```python
from build123d import *

# Parameters (mm, degrees)
EXTRUDE_1_DEPTH = 5
SKETCH_2_W      = 20
SKETCH_2_H      = 40
EXTRUDE_3_DEPTH = 15
FILLET_1_R      = 10


with BuildPart() as part:
    # 草图1 → 凸台-拉伸1 (new body)
    with BuildSketch(Plane(origin=(0, 0, 0), x_dir=(1, 0, 0), z_dir=(0, 1, 0))):
        with BuildLine():
            Line((0, 0), (100, 0))
            Line((100, 0), (100, 112))
            Line((100, 112), (70, 152))
            ThreePointArc((70, 152), (50, 162), (30, 152))
            Line((30, 152), (0, 112))
            Line((0, 112), (0, 0))
        make_face()
    extrude(amount=EXTRUDE_1_DEPTH)

    # 草图2 → 凸台-拉伸3 (add)
    with BuildSketch(Plane.XZ):
        with Locations((90, -20)):
            Rectangle(SKETCH_2_W, SKETCH_2_H)
        with Locations((10, -20)):
            Rectangle(SKETCH_2_W, SKETCH_2_H)
    extrude(amount=EXTRUDE_3_DEPTH)

    # 圆角1
    fillet_1_edges = [part.edges().sort_by_distance(p)[0] for p in [
        (90, -15, 0),
        (10, -15, 0),
    ]]
    fillet(fillet_1_edges, radius=FILLET_1_R)


solid = part.part
```
Here's how the part is built. I have some questions about the finished solid (model axes, mm). A direction names the side the tool comes from. Round coordinates to 2 decimals unless told otherwise and drop trailing zeros. Order: outer loops, then holes, each group sorted by start corner. A loop starts at its lowest first (then second) coordinate and runs counter-clockwise, first axis right, second up. Notation, with made-up numbers: M -20.75,59.25 L -10.75,59.25 A24 ccw -10.75,71.25 Z; hole C 30,77 d10. An arc over 180 degrees is marked long. Answer as CSV lines item,"result".
Item 1: Please list where these lines run through material, in increasing order: L1, parallel to X at y = -13.75, z = -15.5; L2, parallel to Y at x = 64, z = -69; L3, parallel to Z at x = 88, y = -1. Write a range as [from, to].
From the geometry:
L1,"[0, 20], [80, 100]"
L2,"[0, 5]"
L3,"[-40, 0]"
Item 2: Imagine slicing it at C-C on z = -125. List the corners of the cut face in (x, y) for me.
From the geometry:
outline,"M 9.75,0 L 90.25,0 L 90.25,5 L 9.75,5 Z"
Item 3: Which directions (+Z, -Z, +X, -X, +Y, -Y) give clear straight access to the entire face, cutting with the end or side of a thin tool? Please do faces 1 (the flat face through (0, -3, -32)), 2 (the flat face through (10, -7, -40)), 3 (the flat face through (20, -7, -20)).
From the geometry:
face 1,"+Z, -Z, -X, +Y, -Y"
face 2,"-Z, +X, -X, -Y"
face 3,"+Z, -Z, -Y"
Item 4: Imagine slicing it at A-A on y = -1.75. List the corners of the cut face in (x, z) for me.
From the geometry:
outline,"M 0,-40 L 20,-40 L 20,0 L 0,0 Z; M 80,-40 L 100,-40 L 100,0 L 80,0 Z"
Item 5: We'd pull the mould along X, two halves only. Please class faces 4 (the flat face through (100, -3, -32)), 5 (the flat face through (80, -7, -20)), 6 (the cylindrical face through (90.14, -12.15, -3.01)): +X half, -X half, draft (parallel to the pull), parting line (faces both ways), or undercut.
From the geometry:
face 4,"+X half"
face 5,"undercut"
face 6,"draft"
Item 6: For pin 1 (10 mm diameter, centred on x = 12, y = -0.5, fed in from -Z); pin 2 (7.5 mm diameter, centred on x = 9.5, y = -8, fed in from -Z); pin 3 (6 mm diameter, centred on x = 72.5, y = 1, fed in from +Z), each with a flat end and sliding along its axis, tell me the tip position at first contact or that it passes through.
From the geometry:
pin 1,"z = -134.63"
pin 2,"z = -40"
pin 3,"z = 0"
Item 7: Imagine slicing it at D-D on y = -10. List the corners of the cut face in (x, z) for me.
From the geometry:
outline,"M 0,-40 L 20,-40 L 20,-1.34 L 0,-1.34 Z; M 80,-40 L 100,-40 L 100,-1.34 L 80,-1.34 Z"
Item 8: Imagine slicing it at B-B on x = 89.5. List the corners of the cut face in (y, z) for me, and give its area (3 significant figures).
From the geometry:
outline,"M -15,-40 L 0,-40 L 0,-126 L 5,-126 L 5,0 L -5,0 A10 ccw -15,-10 Z"
area,"1,210 mm2"
